from build123d import *

# Parameters (mm, degrees)
SKETCH1_R                = 1.25
BOSS_EXTRUDE1_DEPTH      = 5
BOSS_EXTRUDE2_DEPTH      = 3
BOSS_EXTRUDE2_DEPTH_BACK = 5
SKETCH2_R                = 1.25
FILLET1_R                = 1
FILLET2_R                = 0.5


with BuildPart() as part:
    # Sketch1 → Boss-Extrude1 (new body)
    with BuildSketch(Plane.XY):
        with BuildLine():
            Line((-8.146317829, 1.615581395), (-8.146317829, -8.884418605))
            Line((-8.146317829, -8.884418605), (-9.896317829, -8.884418605))
            Line((-9.896317829, -8.884418605), (-9.896317829, 5.615581395))
            Line((-9.896317829, 5.615581395), (7.103682171, 5.615581395))
            Line((7.103682171, 5.615581395), (7.103682171, -2.238667294))
            ThreePointArc((7.103682171, -2.238667294), (6.103682171, -4.884418605), (7.103682171, -7.530169916))
            Line((7.103682171, -7.530169916), (7.103682171, -8.884418605))
            Line((7.103682171, -8.884418605), (5.353682171, -8.884418605))
            Line((5.353682171, -8.884418605), (5.353682171, 1.615581395))
            Line((5.353682171, 1.615581395), (-8.146317829, 1.615581395))
        make_face()
        with Locations((-7.896317829, 3.615581395)):
            Circle(SKETCH1_R, mode=Mode.SUBTRACT)
        with Locations((5.103682171, 3.615581395)):
            Circle(SKETCH1_R, mode=Mode.SUBTRACT)
    extrude(amount=BOSS_EXTRUDE1_DEPTH)

    # Sketch2 → Boss-Extrude2 (add, two sides: drawn at the far end of the back side and taken through both)
    with BuildSketch(Plane.XY.offset(5).offset(-BOSS_EXTRUDE2_DEPTH_BACK)):
        with Locations((-7.896317829, 3.615581395)):
            Circle(SKETCH2_R)
        with Locations((5.103682171, 3.615581395)):
            Circle(SKETCH2_R)
    extrude(amount=BOSS_EXTRUDE2_DEPTH + BOSS_EXTRUDE2_DEPTH_BACK)

    # Fillet1
    # the kernel refuses this fillet: 1 mm, written as the material it adds along each edge
    with BuildSketch(Plane(origin=(-8.146317829, 1.615581395, 0), x_dir=(1, 0, 0), z_dir=(0, 0, 1)), Plane(origin=(5.353682171, 1.615581395, 0), x_dir=(0, -1, 0), z_dir=(0, 0, 1))) as fillet1_piece_1:
        with BuildLine():
            CenterArc((FILLET1_R, -FILLET1_R), FILLET1_R, 90, 90)
            Line((0, -FILLET1_R), (0, 0))
            Line((0, 0), (FILLET1_R, 0))
        make_face()
    extrude(amount=5)
    # the kernel refuses this fillet: 1 mm, written as the material it takes off along each edge
    with BuildSketch(Plane(origin=(-8.146317829, -8.884418605, -2.5), x_dir=(0, 1, 0), z_dir=(0, 0, 1)), Plane(origin=(-9.896317829, -8.884418605, -2.5), x_dir=(1, 0, 0), z_dir=(0, 0, 1)), Plane(origin=(-9.896317829, 5.615581395, -2.5), x_dir=(0, -1, 0), z_dir=(0, 0, 1)), Plane(origin=(5.353682171, -8.884418605, -2.5), x_dir=(1, 0, 0), z_dir=(0, 0, 1))) as fillet1_2_piece_1:
        with BuildLine():
            CenterArc((FILLET1_R, FILLET1_R), FILLET1_R, 180, 90)
            Line((0, FILLET1_R), (0, 0))
            Line((0, 0), (FILLET1_R, 0))
        make_face()
    extrude(amount=10, mode=Mode.SUBTRACT)
    with BuildSketch(Plane(origin=(7.103682171, 5.615581395, -2.5), x_dir=(0, -1, 0), z_dir=(0, 0, 1))) as fillet1_2_piece_2:
        with BuildLine():
            CenterArc((FILLET1_R, -FILLET1_R), FILLET1_R, 90, 90)
            Line((0, -FILLET1_R), (0, 0))
            Line((0, 0), (FILLET1_R, 0))
        make_face()
    extrude(amount=10, mode=Mode.SUBTRACT)

    # Fillet2
    fillet2_edges = [part.edges().sort_by_distance(p)[0] for p in [
        (-9.146317829, 3.615581395, 5),
        (3.853682171, 3.615581395, 5),
        (-9.146317829, 3.615581395, 8),
        (3.853682171, 3.615581395, 8),
    ]]
    fillet(fillet2_edges, radius=FILLET2_R)


solid = part.part
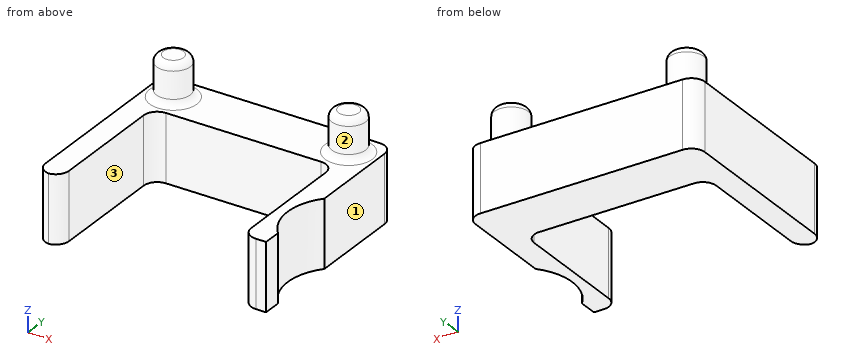
Geometry: final body of the model. Coordinates: model frame, mm. Face numbers are marked on the shaded views. A direction names the side the tool comes from. Round coordinates to 2 decimals unless told otherwise and drop trailing zeros. Order: outer loops, then holes, each group sorted by start corner. A loop starts at its lowest first (then second) coordinate and runs counter-clockwise, first axis right, second up. Notation, with made-up numbers: (88.5, 23) - (131.5, 23) arc R27 ccw to (131.5, 54) - close; hole circle Ø5 at (11, -5.75). An arc over 180 degrees is marked (long way). Write each question's results on one line, items separated by ' | '.
Item 1: Section D-D, the plane x = 1. Return the cut outline in (y, z).
Completed:
outline: (1.62, 0) - (5.62, 0) - (5.62, 5) - (1.62, 5) - close
Item 2: Section C-C, the plane y = -1. Return the cut outline in (x, z), and give its area (3 significant figures).
Completed:
outline: (-9.9, 0) - (-8.15, 0) - (-8.15, 5) - (-9.9, 5) - close; (5.35, 0) - (7.1, 0) - (7.1, 5) - (5.35, 5) - close | area: 17.5 mm^2
Item 3: Section B-B, the plane z = 3. Return the cut outline in (x, y), and give its area (3 significant figures).
Completed:
outline: (-9.9, -7.88) arc R1 ccw to (-9.02, -8.88) arc R1 ccw to (-8.15, -7.88) - (-8.15, 0.62) arc R1 cw to (-7.15, 1.62) - (4.35, 1.62) arc R1 cw to (5.35, 0.62) - (5.35, -7.88) arc R1 ccw to (6.35, -8.88) - (7.1, -8.88) - (7.1, -7.53) arc R4 cw to (7.1, -2.24) - (7.1, 4.62) arc R1 ccw to (6.1, 5.62) - (-8.9, 5.62) arc R1 ccw to (-9.9, 4.62) - close | area: 100 mm^2
Item 4: First-contact query: pin 1 Ø1 at (y, z) = (2.5, 6.5) entering from +X; pin 2 Ø4.5 at (x, y) = (2, 0.5) entering from +Z; pin 3 Ø1.5 at (y, z) = (-5.5, 5.5) entering from +X. Flat tips, straight axial feed; report the tip coordinate or a pass-through.
Completed:
pin 1: x = 6.19 | pin 2: z = 5 | pin 3: x = 6.28
Item 5: Reachability of the marked faces 1, 2 and 3 from +Z, -Z, +X, -X, +Y, -Y: full face, straight path, thin tool, end or side. Return the list, or none.
Completed:
face 1: +Z, -Z, +X, +Y, -Y | face 2: +Z | face 3: +Z, -Z, -Y
Item 6: Material intervals for line 1 along X through (y, z) = (0.25, 2.75); line 2 along X through (y, z) = (-4.75, 1); line 3 along Z through (x, y) = (-4.75, 2.5), sorted ascending. Write a range as [from, to].
Completed:
line 1: [-9.9, -8.15], [5.35, 7.1] | line 2: [-9.9, -8.15], [5.35, 6.11] | line 3: [0, 5]
Item 7: Section A-A, the plane y = -6. Return the cut outline in (x, z), and give its area (3 significant figures).
Completed:
outline: (-9.9, 0) - (-8.15, 0) - (-8.15, 5) - (-9.9, 5) - close; (5.35, 0) - (6.26, 0) - (6.26, 5) - (5.35, 5) - close | area: 13.3 mm^2
